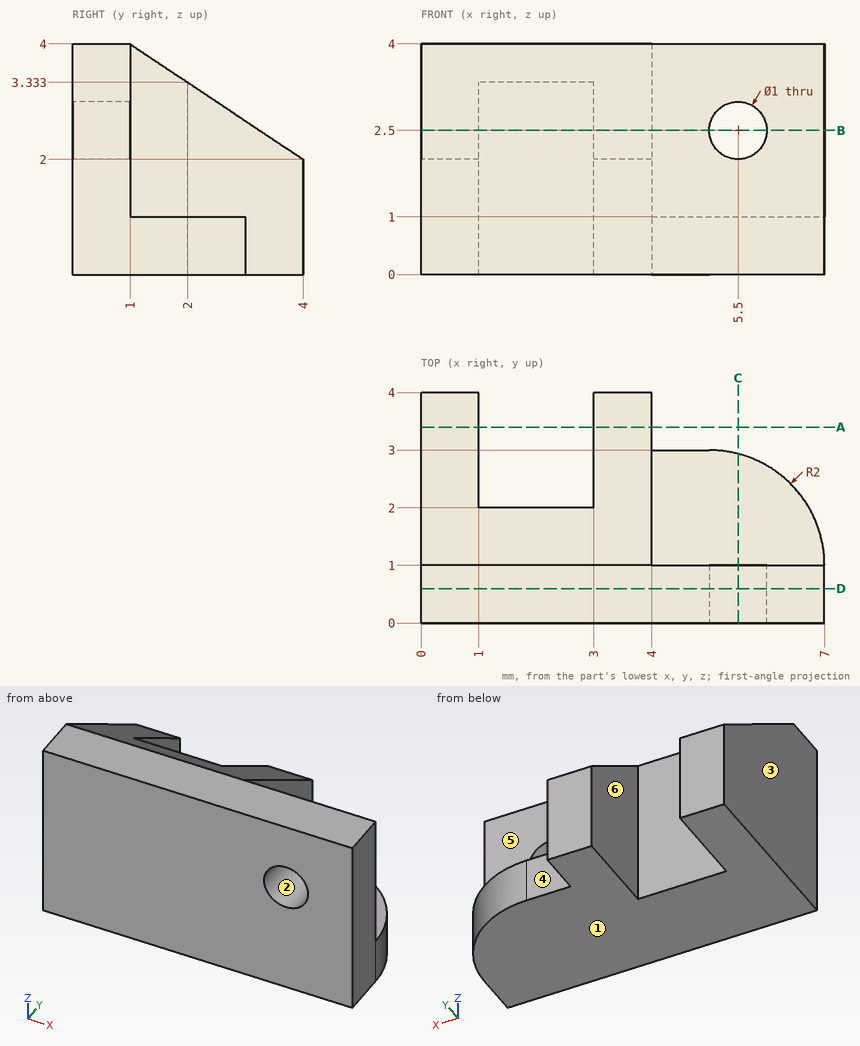
Part print with two shaded views. Sizes in mm from the minimum x, y, z corner. A direction names the side the tool comes from. Give positions to 0.01 mm unless a question says otherwise; leave off trailing zeros. Order: outer loops, then holes, each group sorted by start corner. A loop starts at its lowest first (then second) coordinate and runs counter-clockwise, first axis right, second up. Notation, with made-up numbers: M 39,-6 L 92,-6 A10 ccw 92,4 Z; hole C 23,65 d3. An arc over 180 degrees is marked long. Use one line per item in the form item = value.
1) Two-plate mould, pull along X, no slides. Class the marked faces 1, 2 and 3: released by +X, released by -X, zero draft, split by the parting line, or undercut.
Calculated:
face_1 = zero draft
face_2 = undercut
face_3 = released by -X
2) Saw through at C-C (x = 5.5). Give the cut face in (y, z).
Calculated:
outline = M 0,0 L 2.94,0 L 2.94,1 L 1,1 L 1,2 L 0,2 Z; M 0,3 L 1,3 L 1,4 L 0,4 Z
3) Saw through at A-A (y = 3.4). Give the cut face in (x, z).
Calculated:
outline = M 0,0 L 1,0 L 1,2.4 L 0,2.4 Z; M 3,0 L 4,0 L 4,2.4 L 3,2.4 Z
4) Probe probe 1 along X at (y, z) = (3.65, 1.25); probe 2 along Z at (x, y) = (5.5, 0.7); probe 3 along X at (y, z) = (0.65, 2.5). List the from-to ranges inside material, lowest first.
Calculated:
probe_1 = 0 to 1, 3 to 4
probe_2 = 0 to 2, 3 to 4
probe_3 = 0 to 5, 6 to 7
5) Drop flat-ended pins along their axis: pin 1 (1 mm diameter, centred on y = 3, z = 2.5, fed in from -X); pin 2 (1 mm diameter, centred on x = 2, z = 2, fed in from +Y); pin 3 (2 mm diameter, centred on y = 3.5, z = 2, fed in from +X). Give the stop position or say it passes through.
Calculated:
pin_1 = 0
pin_2 = 2
pin_3 = 4
6) Tool access for the marked faces 4, 5 and 6: list every direction of +Z, -Z, +X, -X, +Y, -Y with a clear straight run to the whole face (end or side of a thin tool).
Calculated:
face_4 = +Z, -Z, +X, +Y
face_5 = +Z, +X, +Y
face_6 = +Z, -Z, +Y
7) Saw through at B-B (z = 2.5). Give the cut face in (x, y), plus the area to 3 significant figures.
Calculated:
outline = M 0,0 L 5,0 L 5,1 L 4,1 L 4,3.25 L 3,3.25 L 3,2 L 1,2 L 1,3.25 L 0,3.25 Z; M 6,0 L 7,0 L 7,1 L 6,1 Z
area = 12.5 mm2
8) Saw through at D-D (y = 0.6). Give the cut face in (x, z).
Calculated:
outline = M 0,0 L 7,0 L 7,4 L 0,4 Z; hole C 5.5,2.5 d1
